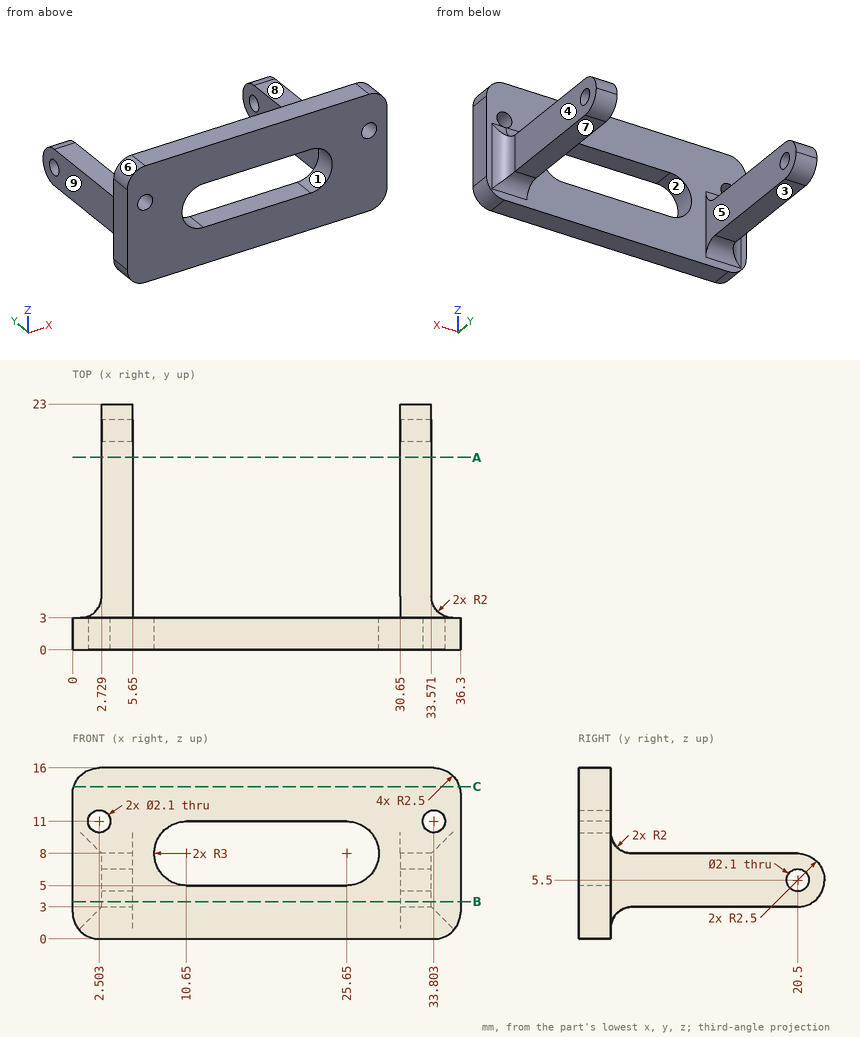
Geometry check sheet. Reference: drawing and pictorial views, mm from the part's lowest x, y, z. A direction names the side the tool comes from. Give positions to 0.01 mm unless a question says otherwise; leave off trailing zeros. Write each loop counter-clockwise with the first axis right and the second up, starting at its lowest first coordinate (ties: lowest second). Pieces come first, ordered by that corner, then holes.
Item 1: Access from +Z, -Z, +X, -X, +Y, -Y to the whole of each face (thin tool, end or side, straight path). Record for the marked faces 5, 6, 7, 8 and 9.
Item 2: Draft check along Z on the marked faces 1, 2, 3 and 4. Enter one of: released by +Z, released by -Z, zero draft, split by the parting line, or undercut.
Item 3: Cross-section at A-A (y = 18). Enter the section's corners in (x, z), and give its area (3 significant figures).
Item 4: Gauge pin test, flat ends, axial feed: pin 1 (4 mm diameter, centred on y = 17, z = 3.5, fed in from +X); pin 2 (1.5 mm diameter, centred on x = 4, y = 11.5, fed in from +Z); pin 3 (4.5 mm diameter, centred on y = 8.5, z = 7.5, fed in from -X). Record the tip position at first contact, or that the pin passes through.
Item 5: Scan lines: L1, parallel to Y at x = 4.4, z = 5.5; L2, parallel to X at y = 12.5, z = 5.5; L3, parallel to Y at x = 35.5, z = 14. Record each from-to range of solid material in increasing order.
Item 6: Cross-section at C-C (z = 14.25). Enter the section's corners in (x, y) (1 decimal).
Item 7: Cross-section at B-B (z = 3.5). Enter the section's corners in (x, y).
Report:
1. face 5: +Z, -Z, +Y
1. face 6: +Z, -X, +Y, -Y
1. face 7: -Z, +X, -X, +Y
1. face 8: +Z, +X, -X, +Y
1. face 9: +Z, -Z, -X, +Y
2. face 1: undercut
2. face 2: undercut
2. face 3: released by -Z
2. face 4: zero draft
3. outline: (2.73, 3) - (5.65, 3) - (5.65, 8) - (2.73, 8) - close; (30.65, 3) - (33.57, 3) - (33.57, 8) - (30.65, 8) - close
3. area: 29.2 mm2
4. pin 1: stops at x = 33.57
4. pin 2: stops at z = 8
4. pin 3: stops at x = 2.73
5. L1: y = 0 to 19.45, 21.55 to 23
5. L2: x = 2.73 to 5.65, 30.65 to 33.57
5. L3: y = 0 to 3
6. outline: (0.1, 0) - (36.2, 0) - (36.2, 3) - (0.1, 3) - close
7. outline: (0, 0) - (36.3, 0) - (36.3, 3) - (35.57, 3) arc R2 cw to (33.57, 5) - (33.57, 22) - (30.65, 22) - (30.65, 3) - (5.65, 3) - (5.65, 22) - (2.73, 22) - (2.73, 5) arc R2 cw to (0.73, 3) - (0, 3) - close
